from build123d import *

# Parameters (mm, degrees)
F3_ANGLE = 180


with BuildPart() as f1:
    # F0 (on Front) → F1 (revolve)
    with BuildSketch(Plane.XZ):
        Polygon((12.75, 150), (15.75, 150), (40.75, 150), (40.75, 175), (12.75, 175), align=None)
        Polygon((6.4, 0), (12.75, 0), (12.75, 13.55), (6.4, 7.2), align=None)
        Polygon((12.75, 0), (15.75, 0), (15.75, 150), (12.75, 150), (12.75, 13.55), align=None)
    revolve(axis=Axis((0, 0, 75), (0, 0, 1)))


with BuildPart() as f1_1:
    # F3: moved
    add(f1.part.rotate(Axis((0, 25.257772, 0), (0, 1, 0)), F3_ANGLE))


solid = f1_1.part
The listing builds one solid part. Answer for the finished solid, in the listing's coordinates (mm). A direction names the side the tool comes from. Coordinates: 2 decimals unless noted, no trailing zeros. Loops run counter-clockwise (first coordinate to the right, second up) from the corner with the lowest first, then second, coordinate; pieces in that order, holes last. Notation, with made-up numbers: (49, -8.75) -> (105, -8.75) arc R7 ccw to (105, -0.75) -> close; hole circle Ø5 at (-7.5, 31.25). An arc over 180 degrees is marked (long way). Answer in a Markdown table with one row per item. Add a question column.
1. For faces 1 (the cylindrical face through (2.764, -12.447, -93.145)), 2 (the flat face through (10, 10, -175)), 3 (the cylindrical face through (2.05, 15.616, -76.05)), determine the directions among +Z, -Z, +X, -X, +Y, -Y from which every point of the face is accessible in a straight line to the end or side of a thin tool.
2. Consider line 1 (Y direction, x = 0, z = -86); line 2 (Y direction, x = 0, z = -3); line 3 (Z direction, x = -15.5, y = -3). Determine where each line is inside the solid, lowest interval first. Write a range as [from, to].
3. Determine the mould class of faces 4 (the conical face through (1.45, -6.55, -7.51)), 5 (the flat face through (18, 1, -150)), 6 (the cylindrical face through (32.338, -24.796, -162.675)), 7 (the cylindrical face through (5.08, -3.89, -3.55)) for opening direction X: +X half, -X half, draft (parallel to the pull), parting line (faces both ways), or undercut.
4. The part is cut by section C-C, the plane z = -132.5. Write down the section's boundary in (x, y).
5. Flat-ended cylindrical pins translate along their axes: P1, Ø3, axis at x = -9, y = 20.5, coming from the +Z side; P2, Ø1.5, axis at x = -4.5, z = -27.5, coming from the -Y side; P3, Ø16.5, axis at x = 0, y = 0, coming from the -Z side. Find the tip coordinate at first contact, or state that the pin passes through.
6. The part is cut by section A-A, the plane y = 0. Write down the section's boundary in (x, z), then the cut area to 3 significant figures.
7. The part is cut by section D-D, the plane x = 23.5. Write down the section's boundary in (y, z), then the cut area to 3 significant figures.
Answer below:
| question | item | result |
|---|---|---|
| 1 | face 1 | -Z |
| 1 | face 2 | -Z, +X, -X, +Y, -Y |
| 1 | face 3 | +Z |
| 2 | line 1 | [-15.75, -12.75], [12.75, 15.75] |
| 2 | line 2 | [-15.75, -6.4], [6.4, 15.75] |
| 2 | line 3 | [-175, -150] |
| 3 | face 4 | undercut |
| 3 | face 5 | draft |
| 3 | face 6 | parting line |
| 3 | face 7 | undercut |
| 4 | outline | circle Ø31.5 at (0, 0); hole circle Ø25.5 at (0, 0) |
| 5 | P1 | z = -150 |
| 5 | P2 | y = -15.3 |
| 5 | P3 | z = -9.05 |
| 6 | outline | (-40.75, -175) -> (-12.75, -175) -> (-12.75, -13.55) -> (-6.4, -7.2) -> (-6.4, 0) -> (-15.75, 0) -> (-15.75, -150) -> (-40.75, -150) -> close; (6.4, -7.2) -> (12.75, -13.55) -> (12.75, -175) -> (40.75, -175) -> (40.75, -150) -> (15.75, -150) -> (15.75, 0) -> (6.4, 0) -> close |
| 6 | area | 2,430 mm2 |
| 7 | outline | (-33.29, -175) -> (33.29, -175) -> (33.29, -150) -> (-33.29, -150) -> close |
| 7 | area | 1,660 mm2 |
